from build123d import *

# Parameters (mm, degrees)
PAD_DEPTH = 615
FILLET_R  = 4


with BuildPart() as part:
    # Sketch → Pad (new body)
    with BuildSketch(Plane.XZ):
        with BuildLine():
            Line((0, 0), (28, 0))
            Line((28, 0), (28, 26))
            ThreePointArc((28, 26), (19.79899, 45.79899), (0, 54))
            Line((0, 54), (0, 0))
        make_face()
    extrude(amount=PAD_DEPTH)

    # Fillet
    fillet_edges = [part.edges().sort_by_distance(p)[0] for p in [
        (0, -307.5, 54),
    ]]
    fillet(fillet_edges, radius=FILLET_R)


solid = part.part
Design review of the part built by this model. Coordinates are the model's own, in mm. Coordinates: 2 decimals unless noted, no trailing zeros. Write each loop counter-clockwise with the first axis right and the second up, starting at its lowest first coordinate (ties: lowest second). Pieces come first, ordered by that corner, then holes. Notation, with made-up numbers: (-17, 78) - (31, 78) arc R23 cw to (31, 107) - close; hole circle Ø2 at (-14.75, -30.75). An arc over 180 degrees is marked (long way). One line per item, written item: value.
1) Add section B-B (x = 11.75). State the section outline as (y, z) points.
Answer sheet:
outline: (-615, 0) - (0, 0) - (0, 51.42) - (-615, 51.42) - close
2) Add section A-A (y = -46). State the section outline as (x, z) points.
Answer sheet:
outline: (0, 0) - (28, 0) - (28, 26) arc R28 ccw to (4.67, 53.61) arc R4 ccw to (0, 49.66) - close
3) To check wall thickness, follow probe 1 along X at (y, z) = (-293, 50); probe 2 along Z at (x, y) = (5, -543); probe 3 along Z at (x, y) = (15.5, -274.5). State the ranges of each line that lie inside material, in increasing order.
Answer sheet:
probe 1: x = 0.01 to 14.42
probe 2: z = 0 to 53.55
probe 3: z = 0 to 49.32
4) Insertion check: pin 1 (8 mm diameter, centred on x = 12, y = -314.5, fed in from +Z); pin 2 (3 mm diameter, centred on x = 21, y = -544.5, fed in from +Z); pin 3 (1.5 mm diameter, centred on x = 19.5, y = -404, fed in from +Z). Each pin has a flat end and moves straight along its axis. Give the tip position at first contact, or say it passes through.
Answer sheet:
pin 1: stops at z = 52.83
pin 2: stops at z = 46.09
pin 3: stops at z = 46.8
5) Add section C-C (z = 38). State the section outline as (x, y) points.
Answer sheet:
outline: (0, -615) - (25.3, -615) - (25.3, 0) - (0, 0) - close
